```python
from build123d import *

# Parameters (mm, degrees)
BOSS_EXTRUDE2_DEPTH = 5
SKETCH5_W           = 5.32214827
SKETCH5_H           = 59.994190195
BOSS_EXTRUDE4_DEPTH = 8.5
BOSS_EXTRUDE5_START = 8.5
BOSS_EXTRUDE5_DEPTH = 8.5
SKETCH7_R           = 1
CUT_EXTRUDE1_DEPTH  = 8.5


with BuildPart() as part:
    # Sketch1 → Boss-Extrude2 (new body)
    with BuildSketch(Plane(origin=(0, 0, 0), x_dir=(1, 0, 0), z_dir=(0, 1, 0))):
        with BuildLine():
            Line((-32.160092199, -30), (-28.617759531, -29.994190195))
            Line((-28.617759531, -29.994190195), (-10.646867834, -29.964716006))
            Line((-10.646867834, -29.964716006), (7.978436277, -23.692711001))
            ThreePointArc((7.978436277, -23.692711001), (12.892303289, -21.419349101), (17.201484904, -18.141359296))
            ThreePointArc((17.201484904, -18.141359296), (25, 0), (17.201484904, 18.141359296))
            ThreePointArc((17.201484904, 18.141359296), (12.892303289, 21.419349101), (7.978436277, 23.692711001))
            Line((7.978436277, 23.692711001), (-10.646867834, 29.964716006))
            Line((-10.646867834, 29.964716006), (-27.981736935, 29.994131783))
            Line((-27.981736935, 29.994131783), (-31.439907801, 30))
            Line((-31.439907801, 30), (-33.939907801, 30))
            Line((-33.939907801, 30), (-33.939907801, -30))
            Line((-33.939907801, -30), (-32.160092199, -30))
        make_face()
    extrude(amount=BOSS_EXTRUDE2_DEPTH)

    # Sketch5 → Boss-Extrude4 (add)
    with BuildSketch(Plane.XZ):
        with Locations((-31.278833666, -0.002904903)):
            Rectangle(SKETCH5_W, SKETCH5_H)
    extrude(amount=BOSS_EXTRUDE4_DEPTH)

    # Sketch6 → Boss-Extrude5 (add)
    with BuildSketch(Plane.XZ.offset(BOSS_EXTRUDE5_START)):
        with BuildLine():
            Line((14.793277017, 15.601568994), (17.201484904, 18.141359296))
            ThreePointArc((17.201484904, 18.141359296), (24.999499268, 0.15822873), (17.429740925, -17.92216871))
            Line((17.429740925, -17.92216871), (15.601568994, -14.793277017))
            ThreePointArc((15.601568994, -14.793277017), (21.492401728, 0.571548738), (14.793277017, 15.601568994))
        make_face()
    extrude(amount=-BOSS_EXTRUDE5_DEPTH)

    # Sketch7 → Cut-Extrude1 (cut)
    with BuildSketch(Plane.XZ):
        with Locations(Location((-6.087958551, 16.72652865, 0), (0, 0, 270))):
            Circle(SKETCH7_R)
        with Locations(Location((0, 0, 0), (0, 0, 270))):
            Circle(SKETCH7_R)
        with Locations(Location((-14.171330366, 9.922872349, 0), (0, 0, 270))):
            Circle(SKETCH7_R)
        with Locations(Location((-16.8, 0, 0), (0, 0, 270))):
            Circle(SKETCH7_R)
        with Locations(Location((-13.352178322, -9.349295913, 0), (0, 0, 270))):
            Circle(SKETCH7_R)
        with Locations(Location((-5.403918265, -14.847143408, 0), (0, 0, 270))):
            Circle(SKETCH7_R)
    extrude(amount=-CUT_EXTRUDE1_DEPTH, mode=Mode.SUBTRACT)

    # Mirror1: part across plane


with BuildPart() as part_1:
    add(part.part)
    add(part.part.mirror(Plane.ZX.offset(-8.5)))


solid = part_1.part
```
The listing builds one solid part. Answer for the finished solid, in the listing's coordinates (mm). A direction names the side the tool comes from. Coordinates: 2 decimals unless noted, no trailing zeros. Write each loop counter-clockwise with the first axis right and the second up, starting at its lowest first coordinate (ties: lowest second). Pieces come first, ordered by that corner, then holes. Notation, with made-up numbers: M -22,37 L 24,37 A24 ccw 24,49 Z; hole C 66,13.25 d3. An arc over 180 degrees is marked long. Use a Markdown table: item, result. Add a question column.
1. Given P1, Ø1, axis at x = -11.5, y = -18, coming from the -Z side; P2, Ø8, axis at x = 2, y = -7.5, coming from the -Z side; P3, Ø6, axis at x = -31.5, y = -10, coming from the +Z side; P4, Ø8, axis at y = -6.5, z = -8.5, coming from the +X side, each flat-ended and moving along its own axis, determine where each tip first touches the part or whether it passes through.
2. Straight lines are drawn through the part: line 1 along X through (y, z) = (2.55, 0); line 2 along Y through (x, z) = (9, 15.5); line 3 along X through (y, z) = (3.75, -0.5) (3 decimals). For each, find the intervals that lie inside material, in ascending order. Write a range as [from, to].
3. Section B-B (y = -1.75) is taken. Give the vertices of the cut face in (x, z), plus the area to 3 significant figures.
4. Which of the six approach directions +Z, -Z, +X, -X, +Y, -Y give full straight-line access (tool end or side, diameter ignored) to faces 4 (the cylindrical face through (21.497, -8.381, 0.335)), 5 (the flat face through (-28.618, -9, 0)), 6 (the flat face through (16.53, -8.62, -16.38))?
5. Section D-D (x = 11) is taken. Give the vertices of the cut face in (y, z).
6. Section C-C (x = 0) is taken. Give the vertices of the cut face in (y, z).
7. Section A-A (z = 0) is taken. Give the vertices of the cut face in (x, y), plus the area to 3 significant figures.
8. For a pull along X with two mould halves and no side action, classify faces 1 (the flat face through (-33.94, -9, 0)), 2 (the cylindrical face through (-15.148, 2.465, 10.14)), 3 (the flat face through (-33, -19, 30)) as +X half, -X half, draft (parallel to the pull), parting line (faces both ways), or undercut.
Data:
| question | item | result |
|---|---|---|
| 1 | P1 | stops at z = -29.97 |
| 1 | P2 | passes through |
| 1 | P3 | stops at z = 29.99 |
| 1 | P4 | stops at x = 24.59 |
| 2 | line 1 | x = [-33.94, -17.8], [-15.8, -1], [1, 25] |
| 2 | line 2 | y = [-22, -17], [0, 5] |
| 2 | line 3 | x = [-33.94, -17.666], [-15.934, -0.866], [0.866, 24.995] |
| 3 | outline | M -33.94,-30 L -28.62,-30 L -28.62,29.99 L -33.94,29.99 Z; M 14.79,15.6 A21.5 cw 15.6,-14.79 L 17.43,-17.92 A25 ccw 17.2,18.14 Z |
| 3 | area | 449 mm2 |
| 4 | face 4 | none |
| 4 | face 5 | +Z, -Z |
| 4 | face 6 | -Z |
| 5 | outline | M -22,-22.45 L -17,-22.45 L -17,22.45 L -22,22.45 Z; M 0,-22.45 L 5,-22.45 L 5,22.45 L 0,22.45 Z |
| 6 | outline | M -22,-26.38 L -17,-26.38 L -17,-1 L -22,-1 Z; M -22,1 L -17,1 L -17,26.38 L -22,26.38 Z; M 0,-26.38 L 5,-26.38 L 5,-1 L 0,-1 Z; M 0,1 L 5,1 L 5,26.38 L 0,26.38 Z |
| 7 | outline | M -33.94,-22 L -17.8,-22 L -17.8,-17 L -28.62,-17 L -28.62,0 L -17.8,0 L -17.8,5 L -33.94,5 Z; M -15.8,-22 L -1,-22 L -1,-17 L -15.8,-17 Z; M -15.8,0 L -1,0 L -1,5 L -15.8,5 Z; M 1,-22 L 25,-22 L 25,5 L 1,5 L 1,0 L 21.5,0 L 21.5,-17 L 1,-17 Z |
| 7 | area | 699 mm2 |
| 8 | face 1 | -X half |
| 8 | face 2 | undercut |
| 8 | face 3 | draft |
